Read the model definition and answer for the solid it produces. Units are mm, in the model's axes. A direction names the side the tool comes from. Give positions to 0.01 mm unless a question says otherwise; leave off trailing zeros. Write each loop counter-clockwise with the first axis right and the second up, starting at its lowest first coordinate (ties: lowest second). Pieces come first, ordered by that corner, then holes. Notation, with made-up numbers: (-32.5, -25.75) -> (7.5, -25.75) arc R5 ccw to (7.5, -17.75) -> close; hole circle Ø2 at (44, -19). An arc over 180 degrees is marked (long way). Use a Markdown table: item, result.
from build123d import *

# Parameters (mm, degrees)
V09_H_BODY102P7X57_FROM_NEW_MANUAL_START = 7
V09_H_BODY102P7X57_FROM_NEW_MANUAL_DEPTH = 51.8
V09_H_FLANGE111P2X65P3_DEPTH7_DEPTH      = 7


with BuildPart() as part:
    # 草图5 → V09_H_body102p7x57_from_new_manual (new body)
    with BuildSketch(Plane.XY.offset(V09_H_BODY102P7X57_FROM_NEW_MANUAL_START)):
        with BuildLine():
            Line((34.15, 8.15), (132.85, 8.15))
            ThreePointArc((132.85, 8.15), (134.264213562, 8.735786438), (134.85, 10.15))
            Line((134.85, 10.15), (134.85, 63.15))
            ThreePointArc((134.85, 63.15), (134.264213562, 64.564213562), (132.85, 65.15))
            Line((132.85, 65.15), (34.15, 65.15))
            ThreePointArc((34.15, 65.15), (32.735786438, 64.564213562), (32.15, 63.15))
            Line((32.15, 63.15), (32.15, 10.15))
            ThreePointArc((32.15, 10.15), (32.735786438, 8.735786438), (34.15, 8.15))
        make_face()
    extrude(amount=V09_H_BODY102P7X57_FROM_NEW_MANUAL_DEPTH)

    # 草图6 → V09_H_flange111p2x65p3_depth7 (add)
    with BuildSketch(Plane.XY):
        with BuildLine():
            Line((30.9, 4), (136.1, 4))
            ThreePointArc((136.1, 4), (138.221320344, 4.878679656), (139.1, 7))
            Line((139.1, 7), (139.1, 66.3))
            ThreePointArc((139.1, 66.3), (138.221320344, 68.421320344), (136.1, 69.3))
            Line((136.1, 69.3), (30.9, 69.3))
            ThreePointArc((30.9, 69.3), (28.778679656, 68.421320344), (27.9, 66.3))
            Line((27.9, 66.3), (27.9, 7))
            ThreePointArc((27.9, 7), (28.778679656, 4.878679656), (30.9, 4))
        make_face()
    extrude(amount=V09_H_FLANGE111P2X65P3_DEPTH7_DEPTH)


solid = part.part
Item 1: Each of these flat-tipped pins is pushed along its axis until it touches: P1, Ø15.5, axis at x = 102.5, z = 44, coming from the +Y side; P2, Ø1, axis at y = 57.5, z = 20, coming from the -X side; P3, Ø4, axis at y = 58.5, z = 21.5, coming from the +X side. Where does it stop, or does it pass through?
Return value:
| item | result |
|---|---|
| P1 | y = 65.15 |
| P2 | x = 32.15 |
| P3 | x = 134.85 |
Item 2: A tool of negligible diameter and unlimited length cuts with its end or side. For faces 1 (the face through (134.85, 36, 33)), 2 (the face through (32.15, 37, 33)), 3 (the face through (79, 8, 7)), from which of +Z, -Z, +X, -X, +Y, -Y can it reach the whole face along a straight path? Write none if from no direction.
Return value:
| item | result |
|---|---|
| face 1 | +Z, +X, +Y, -Y |
| face 2 | +Z, -X, +Y, -Y |
| face 3 | +Z |
Item 3: A cutting plane is placed at B-B (y = 23). Give the vertices of the cut face in (x, z).
Return value:
| item | result |
|---|---|
| outline | (27.9, 0) -> (139.1, 0) -> (139.1, 7) -> (134.85, 7) -> (134.85, 58.8) -> (32.15, 58.8) -> (32.15, 7) -> (27.9, 7) -> close |
Item 4: Straight lines are drawn through the part: line 1 along X through (y, z) = (61, 46.5); line 2 along Y through (x, z) = (69, 17.5). For each, find the intervals that lie inside material, in ascending order. Write a range as [from, to].
Return value:
| item | result |
|---|---|
| line 1 | [32.15, 134.85] |
| line 2 | [8.15, 65.15] |
Item 5: A cutting plane is placed at A-A (x = 88.5). Give the vertices of the cut face in (y, z), then the cut area to 3 significant figures.
Return value:
| item | result |
|---|---|
| outline | (4, 0) -> (69.3, 0) -> (69.3, 7) -> (65.15, 7) -> (65.15, 58.8) -> (8.15, 58.8) -> (8.15, 7) -> (4, 7) -> close |
| area | 3,410 mm^2 |
